Study the drawing (mm; zero at the part's minimum x, y, z) and answer. A direction names the side the tool comes from. Give positions to 0.01 mm unless a question says otherwise; leave off trailing zeros. Write each loop counter-clockwise with the first axis right and the second up, starting at its lowest first coordinate (ties: lowest second). Pieces come first, ordered by that corner, then holes. Notation, with made-up numbers: (18.25, 59.25) -> (29.25, 59.25) arc R25 cw to (29.25, 83.25) -> close; hole circle Ø2 at (-11.75, -28.75). An arc over 180 degrees is marked (long way). Use CSV: the item, a comma, the result in double quotes. Start each with the question number.
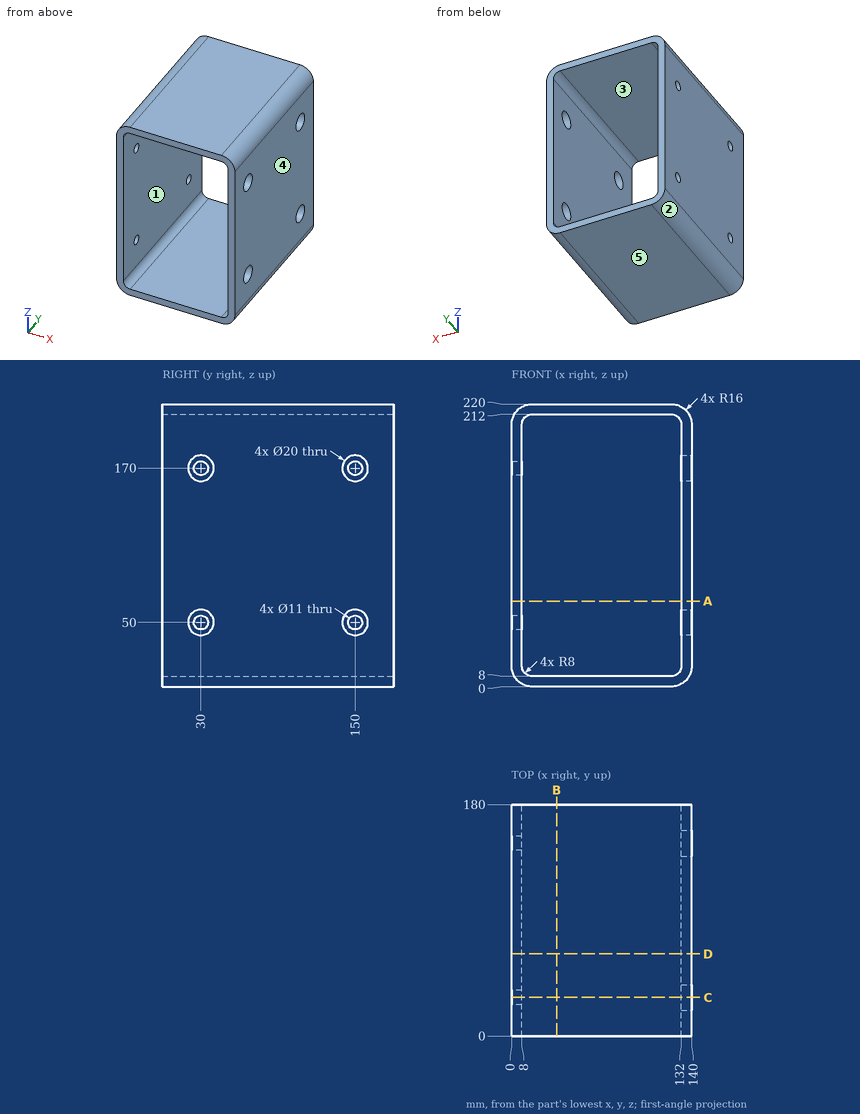
Q1. Section D-D on y = 64 is taken. Give the vertices of the cut face in (x, z), then the cut area to 3 significant figures.
Q2. The mould has two halves that part along X. Classify the marked faces 3, 4 and 5: +X half, -X half, draft (parallel to the pull), parting line (faces both ways), or undercut.
Q3. Flat-ended cylindrical pins translate along their axes: pin 1 Ø12.5 at (y, z) = (30, 50) entering from +X; pin 2 Ø6.5 at (y, z) = (150, 170) entering from -X. Find the tip coordinate at first contact, or state that the pin passes through.
Q4. Section A-A on z = 66.5 is taken. Give the vertices of the cut face in (x, y), then the cut area to 3 significant figures.
Q5. Section B-B on x = 35 is taken. Give the vertices of the cut face in (y, z).
Q6. Section C-C on y = 30 is taken. State how many separate pieces and enclosed holes the cut face has, then the cut area to 3 significant figures.
Q7. For the marked faces 1 and 2, determine the directions among +Z, -Z, +X, -X, +Y, -Y from which every point of the face is accessible in a straight line to the end or side of a thin tool.
Q8. Straight lines are drawn through the part: L1, parallel to Y at x = 2, z = 50; L2, parallel to Y at x = 136, z = 50; L3, parallel to X at y = 49, z = 61.5. For each, find the intervals that lie inside material, in ascending order.
Output:
1,outline,"(0, 16) arc R16 ccw to (16, 0) -> (124, 0) arc R16 ccw to (140, 16) -> (140, 204) arc R16 ccw to (124, 220) -> (16, 220) arc R16 ccw to (0, 204) -> close; hole (8, 16) arc R8 ccw to (16, 8) -> (124, 8) arc R8 ccw to (132, 16) -> (132, 204) arc R8 ccw to (124, 212) -> (16, 212) arc R8 ccw to (8, 204) -> close"
1,area,"5,340 mm²"
2,face 3,"undercut"
2,face 4,"+X half"
2,face 5,"draft"
3,pin 1,"x = 8"
3,pin 2,"through"
4,outline,"(0, 0) -> (8, 0) -> (8, 180) -> (0, 180) -> close; (132, 0) -> (140, 0) -> (140, 180) -> (132, 180) -> close"
4,area,"2,880 mm²"
5,outline,"(0, 0) -> (180, 0) -> (180, 8) -> (0, 8) -> close; (0, 212) -> (180, 212) -> (180, 220) -> (0, 220) -> close"
6,separate pieces,"4"
6,enclosed holes,"0"
6,area,"4,840 mm²"
7,face 1,"+Y, -Y"
7,face 2,"-Z, -X, +Y, -Y"
8,L1,"0 to 24.5, 35.5 to 144.5, 155.5 to 180"
8,L2,"0 to 20, 40 to 140, 160 to 180"
8,L3,"0 to 8, 132 to 140"
